The listing builds one solid part. Answer for the finished solid, in the listing's coordinates (mm). A direction names the side the tool comes from. Round coordinates to 2 decimals unless told otherwise and drop trailing zeros. Order: outer loops, then holes, each group sorted by start corner. A loop starts at its lowest first (then second) coordinate and runs counter-clockwise, first axis right, second up. Notation, with made-up numbers: (10.5, -34) - (65.5, -34) arc R7 cw to (65.5, -29) - close; hole circle Ø3 at (51, 37). An arc over 180 degrees is marked (long way). Write item = value, one per line.
from build123d import *

# Parameters (mm, degrees)
BOSS_EXTRUDE1_DEPTH             = 2.215
BOSS_EXTRUDE3_REACH             = 201.5
BOSS_EXTRUDE3_START             = -1
BOSS_EXTRUDE3_DIRECTION_2_REACH = 3
CUT_EXTRUDE1_DEPTH              = 5.2
CUT_EXTRUDE2_DEPTH              = 0.7
FILLET1_R                       = 2
FILLET2_R                       = 0.8
FILLET4_R                       = 0.2
FILLET3_R                       = 0.5
FILLET5_R                       = 0.3


with BuildPart() as part:
    # Sketch1 → Boss-Extrude1 (new body, symmetric)
    with BuildSketch(Plane(origin=(0, 0, 0), x_dir=(0, 0, -1), z_dir=(1, 0, 0))):
        Polygon((0, 0), (-5.2, -0.325), (-5.2, -6.475), (-1.13, -6.729375), (-1.13, -198.5), (-0.43, -198.5), (-0.43, -174.5), (0, -170.5), align=None)
    extrude(amount=BOSS_EXTRUDE1_DEPTH, both=True)

    # Boss-Extrude3: up to this face of the body (flat: up to its plane)
    boss_extrude3_end = Plane(part.part.faces().sort_by_distance((0, -6.6021875, 3.165))[0])
    # Sketch2 → Boss-Extrude3 (add, up to the picked face)
    with BuildSketch(Plane(origin=(0, 0, 0), x_dir=(1, 0, 0), z_dir=(0, 1, 0)).offset(BOSS_EXTRUDE3_START), mode=Mode.PRIVATE) as boss_extrude3_sk1:
        Polygon((-3.66, 0), (3.66, 0), (3.5, -5.2), (-3.5, -5.2), align=None)
    boss_extrude3_tool1 = split(extrude(boss_extrude3_sk1.sketch, amount=-BOSS_EXTRUDE3_REACH, mode=Mode.PRIVATE), bisect_by=boss_extrude3_end, keep=Keep.BOTH, mode=Mode.PRIVATE)
    add(boss_extrude3_tool1.solids().sort_by_distance((0, -1, 2.580633))[0])

    # Boss-Extrude3 direction 2: up to this face of the body (flat: up to its plane)
    boss_extrude3_direction_2_end = Plane(part.part.faces().sort_by_distance((0, -0.1625, 2.6))[0])
    # Sketch2 → Boss-Extrude3 direction 2 (add, up to the picked face)
    with BuildSketch(Plane(origin=(0, 0, 0), x_dir=(1, 0, 0), z_dir=(0, 1, 0)).offset(BOSS_EXTRUDE3_START), mode=Mode.PRIVATE) as boss_extrude3_direction_2_sk1:
        Polygon((-3.66, 0), (3.66, 0), (3.5, -5.2), (-3.5, -5.2), align=None)
    boss_extrude3_direction_2_tool1 = split(extrude(boss_extrude3_direction_2_sk1.sketch, amount=BOSS_EXTRUDE3_DIRECTION_2_REACH, mode=Mode.PRIVATE), bisect_by=boss_extrude3_direction_2_end, keep=Keep.BOTH, mode=Mode.PRIVATE)
    add(boss_extrude3_direction_2_tool1.solids().sort_by_distance((0, -1, 2.580633))[0])

    # Sketch3 → Cut-Extrude1 (cut)
    with BuildSketch(Plane.XY.offset(5.2)):
        Polygon((-2.4, -2.225), (2.4, -2.225), (2.4, -3.625), (1.375, -3.625), (1.375, -3.075), (-1.375, -3.075), (-1.375, -3.625), (-2.4, -3.625), align=None)
    extrude(amount=-CUT_EXTRUDE1_DEPTH, mode=Mode.SUBTRACT)

    # Sketch5 → Cut-Extrude2 (cut)
    with BuildSketch(Plane.XY.offset(1.13)):
        with BuildLine():
            Line((0.777423831, -197.888711915), (1.6, -194.5))
            Line((1.6, -194.5), (2.215, -178.5))
            Line((2.215, -178.5), (2.215, -198.6))
            Line((2.215, -198.6), (-2.215, -198.6))
            Line((-2.215, -198.6), (-2.215, -178.5))
            Line((-2.215, -178.5), (-1.6, -194.5))
            Line((-1.6, -194.5), (-0.777423831, -197.888711915))
            ThreePointArc((-0.777423831, -197.888711915), (0, -198.5), (0.777423831, -197.888711915))
        make_face()
    extrude(amount=-CUT_EXTRUDE2_DEPTH, mode=Mode.SUBTRACT)

    # Fillet1
    fillet1_edges = [part.edges().sort_by_distance(p)[0] for p in [
        (2.215, -178.5, 0.78),
        (1.6, -194.5, 0.78),
        (-2.215, -178.5, 0.78),
        (-1.6, -194.5, 0.78),
    ]]
    fillet(fillet1_edges, radius=FILLET1_R)

    # Fillet2
    fillet2_edges = [part.edges().sort_by_distance(p)[0] for p in [
        (3.58, -0.1625, 2.6),
        (3.58, -6.6375, 2.6),
        (-3.58, -0.1625, 2.6),
        (-3.58, -6.6375, 2.6),
    ]]
    fillet(fillet2_edges, radius=FILLET2_R)

    # Fillet4
    fillet4_edges = [part.edges().sort_by_distance(p)[0] for p in [
        (1.165077859, -196.291719596, 1.13),
        (1.911348252, -186.399882881, 1.13),
        (-1.911348252, -186.399882881, 1.13),
        (1.590082395, -194.498619822, 1.13),
        (-1.590082395, -194.498619822, 1.13),
        (1.911348252, -186.399882881, 1.13),
        (-1.911348252, -186.399882881, 1.13),
        (2.215, -92.6146875, 1.13),
        (0, -198.5, 1.13),
        (-1.165077859, -196.291719596, 1.13),
        (-2.215, -92.6146875, 1.13),
    ]]
    fillet(fillet4_edges, radius=FILLET4_R)

    # Fillet3
    fillet3_edges = [part.edges().sort_by_distance(p)[0] for p in [
        (0, -6.729375, 1.13),
        (-2.215, -6.7709375, 0.465),
        (2.215, -6.7709375, 0.465),
        (-2.156490258, -6.733040474, 1.071352421),
        (2.156490258, -6.733040474, 1.071352421),
    ]]
    fillet(fillet3_edges, radius=FILLET3_R)

    # Fillet5
    fillet5_edges = [part.edges().sort_by_distance(p)[0] for p in [
        (0, -6.475, 5.2),
        (-3.5, -3.4, 5.2),
        (0, -0.325, 5.2),
        (3.5, -3.4, 5.2),
        (3.266325663, -6.240562729, 5.2),
        (3.266325663, -0.559437271, 5.2),
        (-3.266325663, -0.559437271, 5.2),
        (-3.266325663, -6.240562729, 5.2),
    ]]
    fillet(fillet5_edges, radius=FILLET5_R)


solid = part.part
Q1. Find the intervals of material crossed by line 1 (Y direction, x = 0, z = 0.55) (3 decimals); line 2 (Y direction, x = 2, z = 4.55) (3 decimals); line 3 (X direction, y = -167.5, z = 0.25) (3 decimals), in increasing order. Write a range as from..to.
Model answer:
line_1 = -198.5..-3.075, -2.225..-0.034
line_2 = -6.516..-3.625, -2.225..-0.284
line_3 = -2.215..2.215
Q2. Determine the mould class of faces 1 (the face through (0, -2.225, 3)), 2 (the face through (0, -3.4, 5.2)) for opening direction X: released by +X, released by -X, zero draft, split by the parting line, or undercut.
Model answer:
face_1 = undercut
face_2 = zero draft
Q3. Section B-B on y = -155.5 is taken. Determine the outline of the cut face in (x, z) (3 decimals).
Model answer:
outline = (-2.215, 0) - (2.215, 0) - (2.215, 0.93) arc R0.2 ccw to (2.015, 1.13) - (-2.015, 1.13) arc R0.2 ccw to (-2.215, 0.93) - close
Q4. Section A-A on y = -176.5 is taken. Determine the outline of the cut face in (x, z) (3 decimals), then the cut area to 3 significant figures.
Model answer:
outline = (-2.215, 0.43) - (2.215, 0.43) - (2.215, 0.93) arc R0.2 ccw to (2.015, 1.13) - (-2.015, 1.13) arc R0.2 ccw to (-2.215, 0.93) - close
area = 3.08 mm^2
Q5. For faces 3 (the face through (0, -86, 0)), 4 (the face through (0, -101, 1.13)), 5 (the face through (0, -184, 0.43)), determine the directions among +Z, -Z, +X, -X, +Y, -Y from which every point of the face is accessible in a straight line to the end or side of a thin tool.
Model answer:
face_3 = -Z, +X, -X, +Y, -Y
face_4 = +Z, +X, -X, -Y
face_5 = -Z, +X, -X, -Y
Q6. Flat-ended cylindrical pins translate along their axes: P1, Ø2, axis at x = -0.5, z = 3, coming from the +Y side (3 decimals); P2, Ø1, axis at y = -83.5, z = 0.5, coming from the -X side (3 decimals); P3, Ø1.5, axis at y = -3, z = 3.5, coming from the +X side; P4, Ø2, axis at y = -161, z = 3.5, coming from the -X side. Find the tip coordinate at first contact, or state that the pin passes through.
Model answer:
P1 = -0.125
P2 = -2.215
P3 = 3.58
P4 = through
